Autodesk Inventor part; units mm, degrees
ref_plane "YZ Plane" through (0, 0, 0) normal (1, 0, 0) x (0, 1, 0)
ref_plane "XZ Plane" through (0, 0, 0) normal (0, 1, 0) x (-1, 0, 0)
ref_plane "XY Plane" through (0, 0, 0) normal (0, 0, 1) x (1, 0, 0)
sketch "スケッチ1" plane through (0, 0, 0) normal (1, 0, 0) x (0, 1, 0)
  circle A0 centre (0, 0) radius 10
  circle A1 centre (0, -10) radius 1.35
  circle A2 centre (8.6603, 5) radius 1.35
  circle A3 centre (-8.6603, 5) radius 1.35
  circle A4 centre (0, 0) radius 5
  line L0 (0, 0) -> (0, 50)
  circle A5 centre (0, 50) radius 22.5
  circle A6 centre (0, 0) radius 14
  line L1 (-14, 0) -> (-22.5, 50)
  line L2 (14, 0) -> (22.5, 50)
  line L3 (0, -14) -> (-11.62, -14)
  line L4 (-11.62, -14) -> (-14, 0)
  line L5 (0, -14) -> (11.62, -14)
  line L6 (11.62, -14) -> (14, 0)
  line L7 (0, 20) -> (-17.4, 20)
  line L8 (0, 20) -> (17.4, 20)
  dimension "d0" = 20
  dimension "d1" = 2.7
  dimension "d4" = 360
  dimension "d6" = 10
  dimension "d7" = 50
  dimension "d8" = 45
  dimension "d9" = 28
extrude "押し出し1" add sketch "スケッチ1" along normal blind 4 contours A0 A1 A3 A2 | A6 L6 L4 | A6 L1 L7 L0 | L0 L8 L2 A6 | L6 L5 A6 | A6 L3 L4
sketch "スケッチ2" plane through (0, -17.4, 20) normal (0, 0, 1) x (1, 0, 0)
  line L0 (0, 17.4) -> (30, 17.4)
  circle A0 centre (30, 17.4) radius 22.5
  circle A1 centre (30, 17.4) radius 18.5
  circle A2 centre (30, 17.4) radius 14.25
  circle A3 centre (48.5, 17.4) radius 1.35
  circle A4 centre (20.75, 33.4215) radius 1.35
  circle A5 centre (20.75, 1.3785) radius 1.35
  line L1 (0, 29.02) -> (0, 34.8)
  line L2 (0, 0) -> (0, 5.78)
  line L3 (0, 34.8) -> (0, 0)
  line L4 (4, 29.02) -> (4, 34.8)
  line L5 (4, 34.8) -> (7, 34.8)
  line L6 (7, 34.8) -> (30, 39.9)
  line L7 (4, 0) -> (4, 5.78)
  line L8 (4, 0) -> (7, 0)
  line L9 (7, 0) -> (30, -5.1)
  line L10 (4, 0) -> (0, 0)
  line L11 (0, 34.8) -> (4, 34.8)
  line L12 (0, 0) -> (0, 34.8)
  line L13 (0, 34.8) -> (4, 34.8)
  dimension "d14" = 37
  dimension "d12" = 30
  dimension "d13" = 45
  dimension "d15" = 28.5
  dimension "d16" = 2.7
  dimension "d19" = 360
  dimension "d21" = 3
  dimension "d22" = 3
extrude "押し出し2" add sketch "スケッチ2" along normal blind 4 contours L3 L1 L11 L5 L6 A0 L0 | L0 A0 L9 L8 L10 L2 L3 | A1 A4 A3 A5 | A0 L6 L9
fillet "フィレット1" radius 3 2 edges at (4, 0, 20) (0, 0, 24)
fillet "フィレット2" radius 3 2 edges at (2, -11.62, -14) (2, 11.62, -14)
sketch "スケッチ7" plane through (0, -17.4, 24) normal (0, 0, 1) x (1, 0, 0)
  circle A0 centre (30, 17.4) radius 14.25
  line L0 (30, 17.4) -> (182.95, 17.4)
  line L1 (30, 17.4) -> (182.95, 17.4) construction
  circle A1 centre (182.95, 17.4) radius 3.5
  circle A2 centre (182.95, 17.4) radius 10
  line L2 (182.95, 27.4) -> (50.1556, 27.4)
  arc A3 (30, -5.1) -> (30, 39.9) centre (30, 17.4) ccw
  line L3 (182.95, 27.4) -> (315.7444, 27.4) construction
  line L4 (182.95, 7.4) -> (50.1556, 7.4)
  point P0 (0, 17.4)
  dimension "d55" = 152.95
  dimension "d56" = 0
  dimension "d57" = 7
  dimension "d58" = 20
  dimension "d59" = 180
extrude "押し出し7" add sketch "スケッチ7" against normal blind 4 contours A3 L2 A2 L0 | L0 A2 L4 A3 | A2
sketch "スケッチ8" plane through (0, -17.4, 24) normal (0, 0, 1) x (1, 0, 0)
  circle A0 centre (20.75, 33.4215) radius 1.35
  circle A1 centre (20.75, 33.4215) radius 2.5
  circle A2 centre (48.5, 17.4) radius 1.35
  circle A3 centre (48.5, 17.4) radius 2.5
  circle A4 centre (20.75, 1.3785) radius 1.35
  circle A5 centre (20.75, 1.3785) radius 2.5
  point P0 (0, 17.4)
  dimension "d63" = 5
  dimension "d64" = 5
  dimension "d65" = 5
extrude "押し出し8" cut sketch "スケッチ8" against normal blind 2 contours A0 | A1 | A3 | A4 | A5
fillet "フィレット4" radius 2 1 edges at (50.1556, 10, 22)
sketch "スケッチ10" plane through (0, -17.4, 24) normal (0, 0, 1) x (1, 0, 0)
  arc A0 (182.95, 7.4) -> (182.95, 27.4) centre (182.95, 17.4) ccw
  line L0 (182.95, 27.4) -> (207.95, 27.4)
  line L1 (207.95, 0) -> (44.265, 0)
  arc A1 (30, -5.1) -> (50.1556, 7.4) centre (30, 17.4) ccw
  line L2 (207.95, 27.4) -> (207.95, 0)
  line L3 (207.95, 0) -> (222.95, 0)
  line L4 (222.95, 0) -> (222.95, 30)
  line L5 (222.95, 30) -> (217.95, 30)
  line L6 (217.95, 30) -> (217.95, 7.4)
  line L7 (217.95, 7.4) -> (207.95, 7.4)
  circle A2 centre (182.95, 17.4) radius 3.5
  circle A3 centre (182.95, 17.4) radius 10
  circle A4 centre (30, 17.4) radius 22.5
  line L8 (50.1556, 7.4) -> (182.95, 7.4)
  point P0 (0, 17.4)
  dimension "d75" = 25
  dimension "d76" = 15
  dimension "d77" = 30
  dimension "d78" = 5
extrude "押し出し10" add sketch "スケッチ10" against normal blind 4 contours A0 L0 L2 L1 A1 L8 | L7 L6 L5 L4 L3 L2
fillet "フィレット5" radius 10 1 edges at (207.95, 10, 22)
fillet "フィレット6" radius 2 6 edges at (217.95, 12.6, 22) (222.95, 12.6, 22) (217.95, -10, 22) (207.95, -10, 22) (222.95, -17.4, 22) (44.265, -17.4, 22)
properties part number "motor_holder_2" material "アルミニウム 6061"
Geometry: final body of the model. Coordinates: model frame, mm. A direction names the side the tool comes from. Round coordinates to 2 decimals unless told otherwise and drop trailing zeros. Loops run counter-clockwise (first coordinate to the right, second up) from the corner with the lowest first, then second, coordinate; pieces in that order, holes last. Notation, with made-up numbers: (27.5, -1.75) - (34.5, -1.75) arc R23 ccw to (34.5, 30.25) - close; hole circle Ø8 at (71, 85). An arc over 180 degrees is marked (long way). Write each question's results on one line, items separated by ' | '. Start each with the question number.
1) First-contact query: P1, Ø3, axis at x = 20.75, y = -16.02, coming from the -Z side; P2, Ø1.2, axis at x = 5, z = 21.5, coming from the +Y side; P3, Ø2.5, axis at x = 21.5, y = -15.5, coming from the +Z side. Flat tips, straight axial feed; report the tip coordinate or a pass-through.
2) Cut plane B-B on x = 128. Return loops of the section in (y, z), then the cut area to 3 significant figures.
3) Line query: probe 1 along Y at (x, z) = (20.75, 20.45); probe 2 along X at (y, z) = (-12.5, 1.5); probe 3 along Z at (x, y) = (198, -16). Output: solid intervals per line, ascending. Write a range as [from, to].
4) Cut plane A-A on z = -2. Return loops of the section in (x, y).
5) Cut plane C-C on z = 14.5. Return loops of the section in (x, y) (3 decimals).
6) Access query for faces 4 (the face through (207.95, -4, 22)), 5 (the face through (3, 17.4, 22)), 6 (the face through (22, -17, 22)), 7 (the face through (4, -17.4, 22)), 8 (the face through (87, -5, 24)). Directions: +Z, -Z, +X, -X, +Y, -Y. A direction counts if a zero-diameter tool reaches every point of the face in a straight line with its end or side. Return the directions, or none.
7) Mould query, pull axis X, two halves, no side actions, for faces 1 (the face through (50.81, -0.96, 23.01)), 2 (the face through (1.895, -14.685, 4.028)), 3 (the face through (222.95, -3, 22)). Classes: released by +X, released by -X, zero draft, split by the parting line, or undercut.
Verdict:
1) P1: stops at z = 20 | P2: stops at y = 17.4 | P3: stops at z = 22
2) outline: (-17.4, 20) - (10, 20) - (10, 24) - (-17.4, 24) - close | area: 110 mm2
3) probe 1: y = [-20.45, -17.37], [-14.67, -10.84], [10.84, 14.67], [17.37, 20.45] | probe 2: x = [0, 4] | probe 3: z = [20, 24]
4) outline: (0, -13.66) - (4, -13.66) - (4, -4.58) - (0, -4.58) - close; (0, 4.58) - (4, 4.58) - (4, 13.66) - (0, 13.66) - close
5) outline: (0, -16.465) - (4, -16.465) - (4, 16.465) - (0, 16.465) - close
6) face 4: +Z, -Z, +Y | face 5: +Z, -Z, -X, +Y | face 6: +Z | face 7: +Z, -Z, -X, -Y | face 8: +Z, +X, -X, +Y, -Y
7) face 1: undercut | face 2: zero draft | face 3: released by +X
